The listing builds one solid part. Answer for the finished solid, in the listing's coordinates (mm). Round coordinates to 2 decimals unless told otherwise and drop trailing zeros. Loops run counter-clockwise (first coordinate to the right, second up) from the corner with the lowest first, then second, coordinate; pieces in that order, holes last. Notation, with made-up numbers: (-1, -39.5) - (49, -39.5) arc R25 ccw to (49, -9.5) - close; hole circle Ø1 at (-38, 27.25). An arc over 180 degrees is marked (long way). Write item = value, one per line. Start each with the question number.
1) Given pin 1 Ø10 at (x, z) = (20.5, 38) entering from +Y; pin 2 Ø8 at (x, y) = (11.5, 9) entering from -Z; pin 3 Ø10 at (x, z) = (18, 25) entering from +Y, each flat-ended and moving along its own axis, determine where each tip first touches the part or whether it passes through.
2) Straight lines are drawn through the part: line 1 along Y through (x, z) = (26.75, 5); line 2 along Z through (x, y) = (26.75, 4.5); line 3 along X through (y, z) = (2.75, 69.5) (3 decimals). For each, find the intervals that lie inside material, in ascending order.
3) Section C-C, the plane z = 34 is taken. Determine the outline of the cut face in (x, y) (3 decimals).
4) Section B-B, the plane x = 18.25 is taken. Determine the outline of the cut face in (y, z).
from build123d import *

# Parameters (mm, degrees)
BOSS_EXTRUDE1_DEPTH = 88.9
CHAMFER1_SIZE       = 28.575


with BuildPart() as part:
    # Sketch1 → Boss-Extrude1 (new body)
    with BuildSketch(Plane.XY):
        Polygon((0, 0), (0, 19.558), (28.575, 8.589085199), (28.575, 0), align=None)
    extrude(amount=BOSS_EXTRUDE1_DEPTH)

    # Chamfer1
    chamfer1_edges = [part.edges().sort_by_distance(p)[0] for p in [
        (0, 9.779, 88.9),
        (0, 9.779, 0),
    ]]
    chamfer(chamfer1_edges, length=CHAMFER1_SIZE - 0.0001)  # a hair under: the kernel refuses the full size


solid = part.part
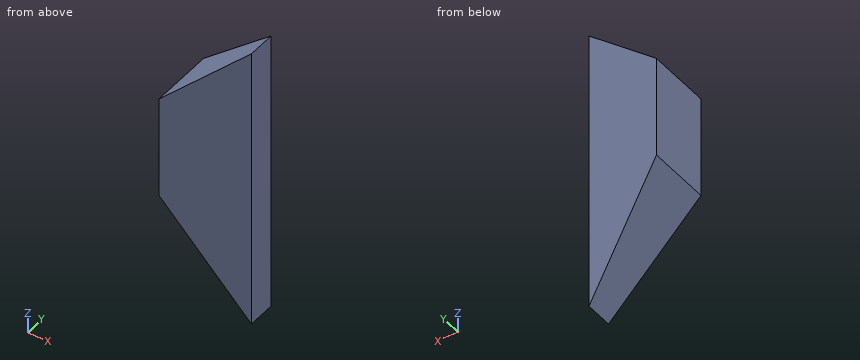
Geometry check:
q1.pin_1 = 13.61
q1.pin_2 = 13.07
q1.pin_3 = 14.57
q2.line_1 = 0 to 9.29
q2.line_2 = 1.82 to 87.08
q2.line_3 = 9.175 to 28.575
q3.outline = (0, 0) - (28.575, 0) - (28.575, 8.589) - (0, 19.558) - close
q4.outline = (0, 10.32) - (12.55, 10.32) - (12.55, 78.58) - (0, 78.58) - close
